Design review of the part built by this model. Coordinates are the model's own, in mm. A direction names the side the tool comes from. Coordinates: 2 decimals unless noted, no trailing zeros. Loops run counter-clockwise (first coordinate to the right, second up) from the corner with the lowest first, then second, coordinate; pieces in that order, holes last.
Q1. Add section A-A on x = -17. Give the boundary of the cut face in (y, z).
Q2. Draft analysis for pull direction Y (two halves, no side actions). For faces 3 (the face through (-1, 0, -1)), 4 (the face through (-39.35, 9.55, -33.55)), 5 (the face through (-7.814, 22.535, -48.479)), 6 (the face through (-41, 13, 29)), state which applies: released by +Y, released by -Y, zero draft, split by the parting line, or undercut.
Q3. Machinability: for faces 1 (the face through (8.286, 9.549, 29.482)), 2 (the face through (-1, 22, 50)), which of the approach directions +Z, -Z, +X, -X, +Y, -Y give a long, thin tool a straight path to every point of the face, cutting with its end or side? Answer none if there is none.
Q4. For P1, Ø14.5, axis at x = 39.5, z = -14.5, coming from the +Y side; P2, Ø6.5, axis at x = 8.18, z = 31.98, coming from the +Y side; P3, Ø1.5, axis at x = 15, z = 37.5, coming from the +Y side, all flat-tipped, find the tip position at first contact; note any pin that passes through.
Q5. Add section D-D on y = 28. Give the boundary of the cut face in (x, z), and give its area (3 significant figures).
Q6. Add section B-B on y = 9.5. Give the number of separate pieces and of enclosed holes in the cut face, and give its area (3 significant figures).
Q7. Wall thickness on probe 1 along Z at (x, y) = (32, 5); probe 2 along X at (y, z) = (3.5, -8); probe 3 along X at (y, z) = (5.5, 40): over which ranges is each line inside the solid? List them lowest first.
Q8. Add section C-C on z = -18. Give the boundary of the cut face in (x, y).
```python
from build123d import *

# Parameters (mm, degrees)
SKETCH1_W           = 122
SKETCH1_H           = 100
BOSS_EXTRUDE1_DEPTH = 3
SKETCH2_W           = 122
SKETCH2_H           = 100
BOSS_EXTRUDE2_DEPTH = 5
SHELL1_T            = -3
SKETCH5_W           = 20
SKETCH5_H           = 2
CUT_EXTRUDE1_DEPTH  = 2.4
SKETCH6_W           = 20
SKETCH6_H           = 2
CUT_EXTRUDE2_DEPTH  = 2.4
SKETCH7_R           = 4
BOSS_EXTRUDE3_DEPTH = 10
SKETCH11_R          = 2.5
CUT_EXTRUDE5_DEPTH  = 7
CUT_EXTRUDE6_DEPTH  = 3
SKETCH13_W          = 18
SKETCH13_H          = 44
BOSS_EXTRUDE5_DEPTH = 3
SKETCH14_W          = 16
SKETCH14_H          = 42
CUT_EXTRUDE7_DEPTH  = 3
FILLET1_R           = 5


with BuildPart() as part:
    # Sketch1 → Boss-Extrude1 (new body)
    with BuildSketch(Plane(origin=(0, 0, 0), x_dir=(1, 0, 0), z_dir=(0, 1, 0))):
        Rectangle(SKETCH1_W, SKETCH1_H)
    extrude(amount=BOSS_EXTRUDE1_DEPTH)



with BuildPart() as body_2:
    # Sketch2 → Boss-Extrude2 (new body)
    with BuildSketch(Plane(origin=(0, 38, 0), x_dir=(1, 0, 0), z_dir=(0, 1, 0))):
        Rectangle(SKETCH2_W, SKETCH2_H)
    extrude(amount=BOSS_EXTRUDE2_DEPTH)


with BuildPart() as part_1:
    add(part.part)

    add(body_2.part)  # loft1 joins it to this body
    # loft from a face of the part (loft1)
    loft([part_1.faces().sort_by_distance((0, 3, 0))[0], part_1.faces().sort_by_distance((0, 38, 0))[0]])

    # Shell1
    shell1_openings = [part_1.faces().sort_by_distance(p)[0] for p in [
        (0, 43, 0),
    ]]
    offset(amount=SHELL1_T, openings=shell1_openings, kind=Kind.INTERSECTION)

    # Sketch5 → Cut-Extrude1 (cut)
    with BuildSketch(Plane.ZY.offset(61)):
        with Locations((0, 40.21846081)):
            Rectangle(SKETCH5_W, SKETCH5_H)
    extrude(amount=-CUT_EXTRUDE1_DEPTH, mode=Mode.SUBTRACT)

    # Sketch6 → Cut-Extrude2 (cut)
    with BuildSketch(Plane(origin=(61, 0, 0), x_dir=(0, 0, -1), z_dir=(1, 0, 0))):
        with Locations((0, 40.177064429)):
            Rectangle(SKETCH6_W, SKETCH6_H)
    extrude(amount=-CUT_EXTRUDE2_DEPTH, mode=Mode.SUBTRACT)

    # Sketch7 → Boss-Extrude3 (add)
    with BuildSketch(Plane(origin=(0, 3, 0), x_dir=(1, 0, 0), z_dir=(0, 1, 0))):
        with Locations(Location((-41.453573848, 34.898312462, 0), (0, 0, 90))):
            Circle(SKETCH7_R)
        with Locations(Location((8.130154931, 34.803413618, 0), (0, 0, 90))):
            Circle(SKETCH7_R)
        with Locations(Location((8.176549105, -31.979822672, 0), (0, 0, 90))):
            Circle(SKETCH7_R)
        with Locations(Location((-41.400089419, -31.94013199, 0), (0, 0, 90))):
            Circle(SKETCH7_R)
    extrude(amount=BOSS_EXTRUDE3_DEPTH)

    # Sketch11 → Cut-Extrude5 (cut)
    with BuildSketch(Plane(origin=(0, 13, 0), x_dir=(1, 0, 0), z_dir=(0, 1, 0))):
        with Locations(Location((-41.400089419, -31.94013199, 0), (0, 0, 270))):
            Circle(SKETCH11_R)
        with Locations(Location((8.176549105, -31.979822672, 0), (0, 0, 270))):
            Circle(SKETCH11_R)
        with Locations(Location((8.130154931, 34.803413618, 0), (0, 0, 270))):
            Circle(SKETCH11_R)
        with Locations(Location((-41.453573848, 34.898312462, 0), (0, 0, 270))):
            Circle(SKETCH11_R)
    extrude(amount=-CUT_EXTRUDE5_DEPTH, mode=Mode.SUBTRACT)

    # Sketch12 → Cut-Extrude6 (cut)
    with BuildSketch(Plane.XY.offset(-47)):
        with BuildLine():
            Line((-21.813500173, 18.623177144), (-11.813500173, 18.623177144))
            ThreePointArc((-11.813500173, 18.623177144), (-7.813500173, 22.623177144), (-11.813500173, 26.623177144))
            Line((-11.813500173, 26.623177144), (-21.813500173, 26.623177144))
            ThreePointArc((-21.813500173, 26.623177144), (-25.813500173, 22.623177144), (-21.813500173, 18.623177144))
        make_face()
    extrude(amount=-CUT_EXTRUDE6_DEPTH, mode=Mode.SUBTRACT)

    # Sketch13 → Boss-Extrude5 (add)
    with BuildSketch(Plane(origin=(0, 3, 0), x_dir=(1, 0, 0), z_dir=(0, 1, 0))):
        with Locations((37.356436199, 16.000571449)):
            Rectangle(SKETCH13_W, SKETCH13_H)
    extrude(amount=BOSS_EXTRUDE5_DEPTH)

    # Sketch14 → Cut-Extrude7 (cut)
    with BuildSketch(Plane(origin=(0, 6, 0), x_dir=(1, 0, 0), z_dir=(0, 1, 0))):
        with Locations((37.356436199, 16.000571449)):
            Rectangle(SKETCH14_W, SKETCH14_H)
    extrude(amount=-CUT_EXTRUDE7_DEPTH, mode=Mode.SUBTRACT)

    # Fillet1
    fillet1_edges = [part_1.edges().sort_by_distance(p)[0] for p in [
        (-41.453573848, 3, -30.898312462),
        (8.130154931, 3, -30.803413618),
        (8.176549105, 3, 35.979822672),
        (-41.400089419, 3, 35.94013199),
    ]]
    fillet(fillet1_edges, radius=FILLET1_R)


solid = part_1.part
```
Entries:
1. outline: (0, -50) - (18.62, -50) - (18.62, -47) - (3, -47) - (3, 47) - (43, 47) - (43, 50) - (0, 50) - close; (26.62, -50) - (43, -50) - (43, -47) - (26.62, -47) - close
2. face 3: released by -Y
2. face 4: zero draft
2. face 5: undercut
2. face 6: released by +Y
3. face 1: +Y
3. face 2: +Z, +X, -X, +Y, -Y
4. P1: stops at y = 6
4. P2: stops at y = 13
4. P3: stops at y = 3.1
5. outline: (-61, -50) - (61, -50) - (61, 50) - (-61, 50) - close; hole (-58, -47) - (58, -47) - (58, 47) - (-58, 47) - close
5. area: 1,300 mm2
6. separate pieces: 5
6. enclosed holes: 5
6. area: 1,420 mm2
7. probe 1: z = -50 to -47, -38 to -37, 5 to 6, 47 to 50
7. probe 2: x = -61 to -58, 28.36 to 29.36, 45.36 to 46.36, 58 to 61
7. probe 3: x = -61 to -58, 58 to 61
8. outline: (-61, 0) - (61, 0) - (61, 43) - (58, 43) - (58, 3) - (46.36, 3) - (46.36, 6) - (45.36, 6) - (45.36, 3) - (29.36, 3) - (29.36, 6) - (28.36, 6) - (28.36, 3) - (-58, 3) - (-58, 43) - (-61, 43) - close
